Design review of the part built by this model. Coordinates are the model's own, in mm. Give positions to 0.01 mm unless a question says otherwise; leave off trailing zeros. Order: outer loops, then holes, each group sorted by start corner. A loop starts at its lowest first (then second) coordinate and runs counter-clockwise, first axis right, second up. Notation, with made-up numbers: (10, 80.25) -> (30, 80.25) arc R16 cw to (30, 88.25) -> close; hole circle Ø3 at (-37, -31.75). An arc over 180 degrees is marked (long way). Return JSON: item names as keys, results as strings.
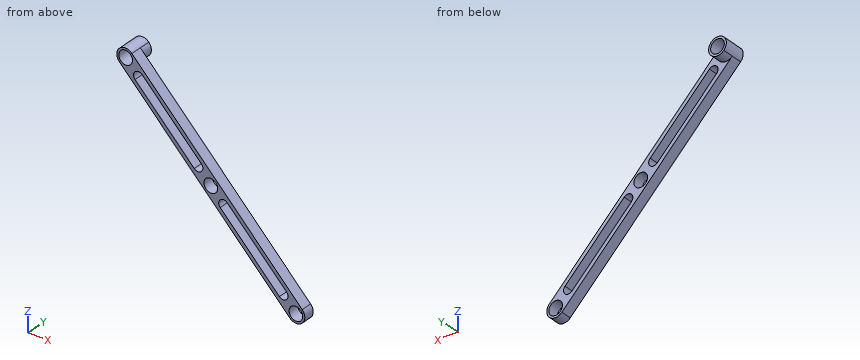
Autodesk Inventor part; units mm, degrees
ref_plane "YZ Plane" through (0, 0, 0) normal (1, 0, 0) x (0, 1, 0)
ref_plane "XZ Plane" through (0, 0, 0) normal (0, 1, 0) x (-1, 0, 0)
ref_plane "XY Plane" through (0, 0, 0) normal (0, 0, 1) x (1, 0, 0)
sketch "Sketch1" plane through (0, 0, 0) normal (0, 1, 0) x (-1, 0, 0)
  circle A0 centre (-56.7045, -56.3864) radius 4.8895
  circle A1 centre (-56.7045, -56.3864) radius 4.8895
  line L0 (-52.2143, -60.8765) -> (69.7375, 61.0754)
  line L1 (60.7573, 70.0556) -> (-61.1946, -51.8963)
  arc A2 (-61.1946, -51.8963) -> (-52.2143, -60.8765) centre (-56.7045, -56.3864) ccw
  arc A3 (69.7375, 61.0754) -> (60.7573, 70.0556) centre (65.2474, 65.5655) ccw
  circle A4 centre (4.2715, 4.5895) radius 4.8895
  circle A5 centre (65.2474, 65.5655) radius 4.8895
  line L2 (7.7289, 8.0469) -> (61.79, 62.1081)
  line L3 (68.7048, 69.0229) -> (69.7375, 70.0556)
  line L4 (-53.2471, -52.929) -> (0.8141, 1.1322) construction
  line L5 (7.7289, 8.0469) -> (61.79, 62.1081) construction
  line L6 (0.8141, 1.1322) -> (-53.2471, -52.929)
  line L7 (-60.1619, -59.8438) -> (-61.1946, -60.8765)
  line L8 (-5.0037, -4.6857) -> (-47.4293, -47.1112) construction
  line L9 (-7.5546, -2.1348) -> (-49.9802, -44.5603)
  line L10 (-44.8784, -49.6621) -> (-2.4529, -7.2365)
  arc A6 (-2.4529, -7.2365) -> (-7.5546, -2.1348) centre (-5.0037, -4.6857) ccw
  arc A7 (-49.9802, -44.5603) -> (-44.8784, -49.6621) centre (-47.4293, -47.1112) ccw
  line L11 (4.2715, 4.5895) -> (-0.2187, 9.0797)
  arc A8 (10.9958, 16.4156) -> (16.0976, 11.3139) centre (13.5467, 13.8648) ccw
  line L12 (10.9958, 16.4156) -> (53.4213, 58.8412)
  line L13 (58.5231, 53.7394) -> (16.0976, 11.3139)
  arc A9 (58.5231, 53.7394) -> (53.4213, 58.8412) centre (55.9722, 56.2903) ccw
  point P0 (0, 0)
  point P1 (29.6663, 4.6577)
  point P2 (-26.2165, -25.8984)
  dimension "d0" = 172.466
  dimension "d1" = 12.7
  dimension "d2" = 9.779
  dimension "d3" = 9.779
  dimension "d4" = 9.779
extrude "Extrusion1" add sketch "Sketch1" along normal blind 7.62 contours A0 L6 A7 L10 A6 A4 L2 A8 L13 A9 A5 L3 A3 L0 A2 L7 | A0 L7 A2 L1 L11 A4 L6 A6 L9 A7 | L1 A3 L3 A5 L2 A9 L12 A8 A4 L11
sketch "Sketch2" plane through (0, 7.62, 0) normal (0, 1, 0) x (1, 0, 0)
  line L0 (-60.7573, -70.0556) -> (61.1946, 51.8963)
  arc A0 (61.1946, 51.8963) -> (52.2143, 60.8765) centre (56.7045, 56.3864) ccw
  line L1 (52.2143, 60.8765) -> (-69.7375, -61.0754)
  arc A1 (-69.7375, -61.0754) -> (-60.7573, -70.0556) centre (-65.2474, -65.5655) ccw
  arc A2 (-58.5231, -53.7394) -> (-53.4213, -58.8412) centre (-55.9722, -56.2903) ccw
  line L2 (-58.5231, -53.7394) -> (-16.0976, -11.3139)
  arc A3 (-10.9958, -16.4156) -> (-16.0976, -11.3139) centre (-13.5467, -13.8648) ccw
  line L3 (-10.9958, -16.4156) -> (-53.4213, -58.8412)
  circle A4 centre (-65.2474, -65.5655) radius 4.8895
  circle A5 centre (-4.2715, -4.5895) radius 4.8895
  circle A6 centre (56.7045, 56.3864) radius 4.8895
  arc A7 (49.9802, 44.5603) -> (44.8784, 49.6621) centre (47.4293, 47.1112) ccw
  line L4 (49.9802, 44.5603) -> (7.5546, 2.1348)
  arc A8 (2.4529, 7.2365) -> (7.5546, 2.1348) centre (5.0037, 4.6857) ccw
  line L5 (2.4529, 7.2365) -> (44.8784, 49.6621)
  circle A9 centre (-65.2474, -65.5655) radius 6.35
  point P0 (0, 0)
extrude "Extrusion2" add sketch "Sketch2" along normal blind 7.62 contours A1 A9
properties part number "Bump Arm"
Item 1: Wall thickness on L1, parallel to Y at x = 2.5, z = 1; L2, parallel to Z at x = 45, y = 3.5; L3, parallel to Z at x = -51.5, y = 2.5: over which ranges is each line inside the solid? List them lowest first. Write a range as [from, to].
Result set:
{"L1": "y = [0, 7.62]", "L2": "z = [-53.66, -49.78], [-39.58, -35.7]", "L3": "z = [42.84, 46.72], [56.92, 60.8]"}
Item 2: Add section C-C (y = 5.5). Give the number of separate pieces and of enclosed holes in the cut face, plus the area to 3 significant figures.
Result set:
{"separate pieces": "1", "enclosed holes": "5", "area": "1,140 mm^2"}
Item 3: Add section D-D (y = 13.5). Give the boundary of the cut face in (x, z).
Result set:
{"outline": "circle Ø12.7 at (-65.25, 65.57); hole circle Ø9.78 at (-65.25, 65.57)"}
Item 4: For pin 1 (11 mm diameter, centred on x = 56.7, z = -56.39, fed in from +Y); pin 2 (8 mm diameter, centred on y = 6.5, z = 6.5, fed in from -X); pin 3 (3 mm diameter, centred on x = -16, y = 4, fed in from +Z), all flat-tipped, find the tip position at first contact; note any pin that passes through.
Result set:
{"pin 1": "stops at y = 7.62", "pin 2": "stops at x = -19.16", "pin 3": "stops at z = 26.8"}
Item 5: Add section B-B (z = -16). Give the boundary of the cut face in (x, y).
Result set:
{"outline": "(7.34, 0) -> (11.22, 0) -> (11.22, 7.62) -> (7.34, 7.62) -> close; (21.42, 0) -> (25.3, 0) -> (25.3, 7.62) -> (21.42, 7.62) -> close"}
Item 6: Add section A-A (x = 5.5). Give the boundary of the cut face in (y, z), plus the area to 3 significant figures.
Result set:
{"outline": "(0, -14.16) -> (7.62, -14.16) -> (7.62, -10.28) -> (0, -10.28) -> close; (0, -1.11) -> (7.62, -1.11) -> (7.62, 3.8) -> (0, 3.8) -> close", "area": "67.0 mm^2"}
